Design review of the part built by this model. Coordinates are the model's own, in mm. Face numbers are marked on the shaded views. A direction names the side the tool comes from. Give positions to 0.01 mm unless a question says otherwise; leave off trailing zeros. Loops run counter-clockwise (first coordinate to the right, second up) from the corner with the lowest first, then second, coordinate; pieces in that order, holes last.
from build123d import *

# Parameters (mm, degrees)
F0_W     = 1.6002
F0_H     = 1.6002
F1_DEPTH = 11.811
F2_R     = 0.508
F3_DEPTH = 11.0871
F5_D     = 1.143
F5_DEPTH = 4.572
F5_TIP   = 0.3433918438


with BuildPart() as f1:
    # F0 (on Top) → F1 (new body)
    with BuildSketch(Plane.XY):
        Rectangle(F0_W, F0_H)
    extrude(amount=F1_DEPTH)

    # F2 (on face) → F3 (join)
    with BuildSketch(Plane.XZ.offset(0.8001)):
        with Locations((0, 10.795)):
            Circle(F2_R)
    extrude(amount=F3_DEPTH)

    # F5
    with Locations(Plane(origin=(0, 0, 0), x_dir=(1, 0, 0), z_dir=(0, 0, -1))):
        with Locations((0, 0)):
            Hole(F5_D / 2, depth=F5_DEPTH)
            with Locations((0, 0, -(F5_DEPTH + F5_TIP / 2))):  # 118° drill point
                Cone(0, F5_D / 2, F5_TIP, mode=Mode.SUBTRACT)


solid = f1.part
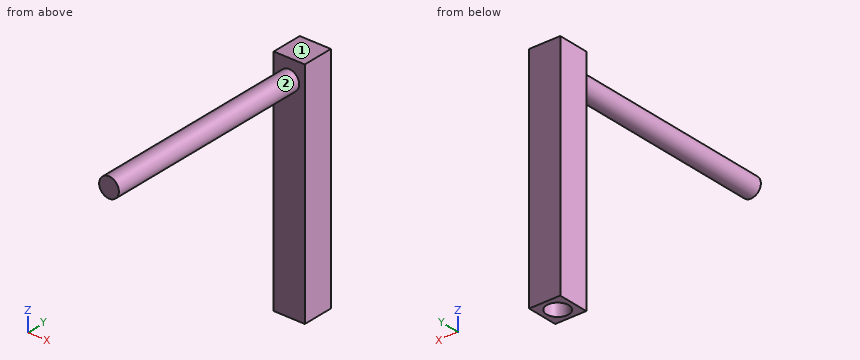
Q1. Take a section at C-C (y = -5.25). Give the boundary of the cut face in (x, z) (3 decimals).
Results:
outline: circle Ø1.016 at (0, 10.795)
Q2. Wall thickness on line 1 (Y direction, x = 0, z = 1.8); line 2 (Y direction, x = 0.25, z = 2); line 3 (Y direction, x = -0.45, z = 5.5): over which ranges is each line inside the solid? List them lowest first.
Results:
line 1: y = -0.8 to -0.57, 0.57 to 0.8
line 2: y = -0.8 to -0.51, 0.51 to 0.8
line 3: y = -0.8 to 0.8
Q3. Tool access review of the marked faces 1 and 2: name each direction out of +Z, -Z, +X, -X, +Y, -Y from which nothing blocks a thin tool from reaching the whole face with its end or side.
Results:
face 1: +Z, +X, -X, +Y, -Y
face 2: -Y
Q4. Take a section at B-B (z = 6). Give the boundary of the cut face in (x, y), plus the area to 3 significant figures.
Results:
outline: (-0.8, -0.8) - (0.8, -0.8) - (0.8, 0.8) - (-0.8, 0.8) - close
area: 2.56 mm2
Q5. Take a section at A-A (z = 1.25). Give the boundary of the cut face in (x, y).
Results:
outline: (-0.8, -0.8) - (0.8, -0.8) - (0.8, 0.8) - (-0.8, 0.8) - close; hole circle Ø1.14 at (0, 0)
Q6. Insertion check: pin 1 (0.7 mm diameter, centred on x = 0, y = 0, fed in from -Z). The pin has a flat end and moves straight along its axis. Give the tip position at first contact, or say it passes through.
Results:
pin 1: stops at z = 4.71
